from build123d import *

# Parameters (mm, degrees)
F0_R     = 38.1
F1_DEPTH = 88.9
F3_D     = 12.7
F5_D     = 19.05


with BuildPart() as f1:
    # F0 (on Top) → F1 (new body)
    with BuildSketch(Plane.XY):
        Circle(F0_R)
    extrude(amount=F1_DEPTH)

    # F3 (through all)
    with Locations(Plane(origin=(0, 0, 0), x_dir=(1, 0, 0), z_dir=(0, 0, -1))):
        with Locations((0, 0)):
            Hole(F3_D / 2)

    # F5 (through all)
    with Locations(Plane(origin=(0, 0, 0), x_dir=(1, 0, 0), z_dir=(0, 0, -1))):
        with Locations((-22.86, 0), (-11.43, -19.797341), (11.43, -19.797341), (22.86, 0), (11.43, 19.797341), (-11.43, 19.797341)):
            Hole(F5_D / 2)


solid = f1.part
The model under review builds one solid part; all positions refer to its coordinate system, in mm. Coordinates: 2 decimals unless noted, no trailing zeros. Write each loop counter-clockwise with the first axis right and the second up, starting at its lowest first coordinate (ties: lowest second). Pieces come first, ordered by that corner, then holes. Notation, with made-up numbers: (59.5, 86) -> (98.5, 86) arc R18 ccw to (98.5, 92) -> close; hole circle Ø3 at (4, 79.25). An arc over 180 degrees is marked (long way). Answer in a Markdown table with one row per item.
1. Clearance check with flat-ended pins moving along their axes: pin 1 Ø1.5 at (x, z) = (1.5, 33) entering from +Y; pin 2 Ø5 at (x, z) = (2, 21.5) entering from -Y; pin 3 Ø1.5 at (x, z) = (21, 14.5) entering from +Y. State where each tip first meets the part, or that it passes through.
Answers below:
| item | result |
|---|---|
| pin 1 | stops at y = 38.09 |
| pin 2 | stops at y = -38.1 |
| pin 3 | stops at y = 32.27 |
2. We need section C-C, the plane y = 1.5. State the section outline as (x, z) points.
Answers below:
| item | result |
|---|---|
| outline | (-38.07, 0) -> (-32.27, 0) -> (-32.27, 88.9) -> (-38.07, 88.9) -> close; (-13.45, 0) -> (-6.17, 0) -> (-6.17, 88.9) -> (-13.45, 88.9) -> close; (6.17, 0) -> (13.45, 0) -> (13.45, 88.9) -> (6.17, 88.9) -> close; (32.27, 0) -> (38.07, 0) -> (38.07, 88.9) -> (32.27, 88.9) -> close |
3. Draft analysis for pull direction X (two halves, no side actions). For faces 1 (the flat face through (8, 1, 88.9)), 2 (the cylindrical face through (-30.235, -23.183, 43.828)), 3 (the cylindrical face through (1.38, 6.2, 45.07)), state which applies: +X half, -X half, draft (parallel to the pull), parting line (faces both ways), or undercut.
Answers below:
| item | result |
|---|---|
| face 1 | draft |
| face 2 | parting line |
| face 3 | undercut |
4. We need section D-D, the plane x = 22.86. State the section outline as (y, z) points (3 decimals), and give its area (3 significant figures).
Answers below:
| item | result |
|---|---|
| outline | (-30.48, 0) -> (-9.525, 0) -> (-9.525, 88.9) -> (-30.48, 88.9) -> close; (9.525, 0) -> (30.48, 0) -> (30.48, 88.9) -> (9.525, 88.9) -> close |
| area | 3,730 mm^2 |
5. We need section B-B, the plane x = -11.43. State the section outline as (y, z) points, and give its area (3 significant figures).
Answers below:
| item | result |
|---|---|
| outline | (-36.35, 0) -> (-29.32, 0) -> (-29.32, 88.9) -> (-36.35, 88.9) -> close; (-10.27, 0) -> (10.27, 0) -> (10.27, 88.9) -> (-10.27, 88.9) -> close; (29.32, 0) -> (36.35, 0) -> (36.35, 88.9) -> (29.32, 88.9) -> close |
| area | 3,080 mm^2 |
6. Wall thickness on probe 1 along X at (y, z) = (-17.5, 29); probe 2 along X at (y, z) = (-12, 8); probe 3 along Y at (x, z) = (0, 72): over which ranges is each line inside the solid? List them lowest first. Write a range as [from, to].
Answers below:
| item | result |
|---|---|
| probe 1 | x = [-33.84, -20.67], [-2.19, 2.19], [20.67, 33.84] |
| probe 2 | x = [-36.16, -16.9], [-5.96, 5.96], [16.9, 36.16] |
| probe 3 | y = [-38.1, -6.35], [6.35, 38.1] |
7. We need section A-A, the plane y = -22. State the section outline as (x, z) points, and give its area (3 significant figures).
Answers below:
| item | result |
|---|---|
| outline | (-31.11, 0) -> (-20.7, 0) -> (-20.7, 88.9) -> (-31.11, 88.9) -> close; (-2.16, 0) -> (2.16, 0) -> (2.16, 88.9) -> (-2.16, 88.9) -> close; (20.7, 0) -> (31.11, 0) -> (31.11, 88.9) -> (20.7, 88.9) -> close |
| area | 2,240 mm^2 |
